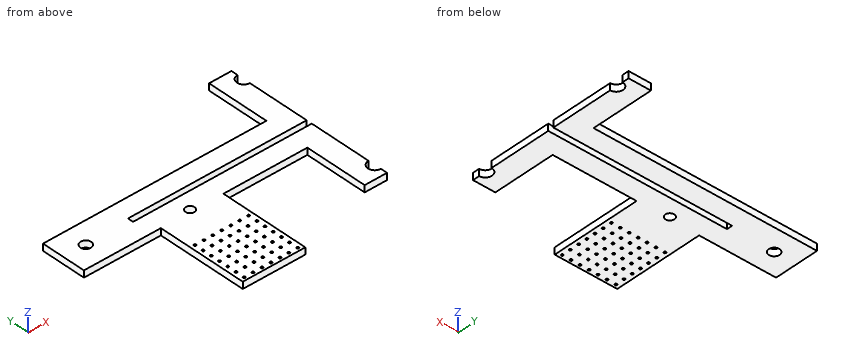
from build123d import *

# Parameters (mm, degrees)
SKETCH1_R           = 1.2
BOSS_EXTRUDE1_DEPTH = 1.5
CUT_EXTRUDE2_DEPTH  = 40
SKETCH2_R           = 0.25
CUT_EXTRUDE4_DEPTH  = 1.5
SKETCH4_R           = 1
CUT_EXTRUDE5_DEPTH  = 1.5


with BuildPart() as part:
    # Sketch1 → Boss-Extrude1 (new body)
    with BuildSketch(Plane.XY):
        with BuildLine():
            ThreePointArc((50, -17.5), (48.5, -16), (50, -14.5))
            Line((50, -14.5), (50, 14.5))
            ThreePointArc((50, 14.5), (48.5, 16), (50, 17.5))
            Line((50, 17.5), (50, 19))
            Line((50, 19), (45, 19))
            Line((45, 19), (45, 5))
            Line((45, 5), (-5, 5))
            Line((-5, 5), (-5, 0))
            Line((-5, 0), (-5, -5))
            Line((-5, -5), (12.22, -5))
            Line((12.22, -5), (12.22, -25))
            Line((12.22, -25), (19.22, -25))
            Line((19.22, -25), (26.22, -25))
            Line((26.22, -25), (26.22, -5))
            Line((26.22, -5), (45, -5))
            Line((45, -5), (45, -19))
            Line((45, -19), (50, -19))
            Line((50, -19), (50, -17.5))
        make_face()
        Circle(SKETCH1_R, mode=Mode.SUBTRACT)
    extrude(amount=BOSS_EXTRUDE1_DEPTH)

    # Sketch3 → Cut-Extrude2 (cut)
    with BuildSketch(Plane(origin=(50, 0, 0), x_dir=(0, 0, -1), z_dir=(1, 0, 0))):
        Polygon((0, 0), (0, -0.625), (-1.5, -0.625), (-1.5, 0.625), (0, 0.625), align=None)
    extrude(amount=-CUT_EXTRUDE2_DEPTH, mode=Mode.SUBTRACT)

    # Sketch2 → Cut-Extrude4 (cut)
    with BuildSketch(Plane.XY.offset(1.5)):
        with Locations((21.22, -24.25)):
            Circle(SKETCH2_R)
        with Locations((19.22, -20.25)):
            Circle(SKETCH2_R)
        with Locations((21.22, -20.25)):
            Circle(SKETCH2_R)
        with Locations((23.22, -20.25)):
            Circle(SKETCH2_R)
        with Locations((23.22, -24.25)):
            Circle(SKETCH2_R)
        with Locations((25.22, -20.25)):
            Circle(SKETCH2_R)
        with Locations((25.22, -18.25)):
            Circle(SKETCH2_R)
        with Locations((23.22, -18.25)):
            Circle(SKETCH2_R)
        with Locations((23.22, -16.25)):
            Circle(SKETCH2_R)
        with Locations((15.22, -24.25)):
            Circle(SKETCH2_R)
        with Locations((21.22, -22.25)):
            Circle(SKETCH2_R)
        with Locations((19.22, -24.25)):
            Circle(SKETCH2_R)
        with Locations((19.22, -22.25)):
            Circle(SKETCH2_R)
        with Locations((19.22, -18.25)):
            Circle(SKETCH2_R)
        with Locations((19.22, -16.25)):
            Circle(SKETCH2_R)
        with Locations((19.22, -14.25)):
            Circle(SKETCH2_R)
        with Locations((19.22, -12.25)):
            Circle(SKETCH2_R)
        with Locations((21.22, -12.25)):
            Circle(SKETCH2_R)
        with Locations((21.22, -14.25)):
            Circle(SKETCH2_R)
        with Locations((21.22, -16.25)):
            Circle(SKETCH2_R)
        with Locations((21.22, -18.25)):
            Circle(SKETCH2_R)
        with Locations((23.22, -22.25)):
            Circle(SKETCH2_R)
        with Locations((25.22, -24.25)):
            Circle(SKETCH2_R)
        with Locations((25.22, -22.25)):
            Circle(SKETCH2_R)
        with Locations((25.22, -16.25)):
            Circle(SKETCH2_R)
        with Locations((23.22, -12.25)):
            Circle(SKETCH2_R)
        with Locations((25.22, -12.25)):
            Circle(SKETCH2_R)
        with Locations((23.22, -14.25)):
            Circle(SKETCH2_R)
        with Locations((25.22, -14.25)):
            Circle(SKETCH2_R)
        with Locations((17.22, -24.25)):
            Circle(SKETCH2_R)
        with Locations((17.22, -22.25)):
            Circle(SKETCH2_R)
        with Locations((17.22, -20.25)):
            Circle(SKETCH2_R)
        with Locations((17.22, -18.25)):
            Circle(SKETCH2_R)
        with Locations((17.22, -16.25)):
            Circle(SKETCH2_R)
        with Locations((17.22, -14.25)):
            Circle(SKETCH2_R)
        with Locations((17.22, -12.25)):
            Circle(SKETCH2_R)
        with Locations((15.22, -22.25)):
            Circle(SKETCH2_R)
        with Locations((15.22, -20.25)):
            Circle(SKETCH2_R)
        with Locations((15.22, -18.25)):
            Circle(SKETCH2_R)
        with Locations((15.22, -16.25)):
            Circle(SKETCH2_R)
        with Locations((15.22, -14.25)):
            Circle(SKETCH2_R)
        with Locations((15.22, -12.25)):
            Circle(SKETCH2_R)
        with Locations((13.22, -12.25)):
            Circle(SKETCH2_R)
        with Locations((13.22, -14.25)):
            Circle(SKETCH2_R)
        with Locations((13.22, -16.25)):
            Circle(SKETCH2_R)
        with Locations((13.22, -18.25)):
            Circle(SKETCH2_R)
        with Locations((13.22, -20.25)):
            Circle(SKETCH2_R)
        with Locations((13.22, -22.25)):
            Circle(SKETCH2_R)
        with Locations((13.22, -24.25)):
            Circle(SKETCH2_R)
    extrude(amount=-CUT_EXTRUDE4_DEPTH, mode=Mode.SUBTRACT)

    # Sketch4 → Cut-Extrude5 (cut)
    with BuildSketch(Plane.XY.offset(1.5)):
        with Locations((19.22, -4.5)):
            Circle(SKETCH4_R)
    extrude(amount=-CUT_EXTRUDE5_DEPTH, mode=Mode.SUBTRACT)


solid = part.part
For this review, take the finished solid that the model builds, in its own axes (mm). Round coordinates to 2 decimals unless told otherwise and drop trailing zeros. Write each loop counter-clockwise with the first axis right and the second up, starting at its lowest first coordinate (ties: lowest second). Pieces come first, ordered by that corner, then holes. Notation, with made-up numbers: (62.25, 50.25) -> (72.25, 50.25) arc R26 cw to (72.25, 74.25) -> close; hole circle Ø1 at (6.25, -37). An arc over 180 degrees is marked (long way). Use CSV: the item, a comma, the result in double quotes.
(1) Consider section A-A, the plane x = 0. Give the boundary of the cut face in (y, z), plus the area to 3 significant figures.
Computed values:
outline,"(-5, 0) -> (-1.2, 0) -> (-1.2, 1.5) -> (-5, 1.5) -> close; (1.2, 0) -> (5, 0) -> (5, 1.5) -> (1.2, 1.5) -> close"
area,"11.4 mm²"
(2) Clearance check with flat-ended pins moving along their axes: P1, Ø0.8, axis at x = 23.5, z = 1, coming from the +Y side; P2, Ø0.8, axis at x = 6, z = 1, coming from the -Y side. State where each tip first meets the part, or that it passes through.
Computed values:
P1,"y = 5"
P2,"y = -5"
(3) Consider section C-C, the plane z = 0.8. Give the number of separate pieces and of enclosed holes in the cut face, plus the area to 3 significant figures.
Computed values:
separate pieces,"1"
enclosed holes,"51"
area,"896 mm²"
(4) Consider section B-B, the plane y = 0. Give the boundary of the cut face in (x, z), plus the area to 3 significant figures.
Computed values:
outline,"(-5, 0) -> (-1.2, 0) -> (-1.2, 1.5) -> (-5, 1.5) -> close; (1.2, 0) -> (10, 0) -> (10, 1.5) -> (1.2, 1.5) -> close"
area,"18.9 mm²"
(5) To check wall thickness, follow L1, parallel to Y at x = 46, z = 0.95 (3 decimals); L2, parallel to X at y = -10.5, z = 0.25; L3, parallel to X at y = 8.5, z = 0.15. State the ranges of each line that lie inside material, in increasing order. Write a range as [from, to].
Computed values:
L1,"[-19, -0.625], [0.625, 19]"
L2,"[12.22, 26.22], [45, 50]"
L3,"[45, 50]"
